from build123d import *

# Parameters (mm, degrees)
SKETCH_2_R          = 3
EXTRUDE_1_DEPTH     = 4
SKETCH_3_R          = 2
EXTRUDE_2_DEPTH     = 3
SKETCH_4_R          = 1
CUT_EXTRUDE_1_DEPTH = 10.110433579
SKETCH_5_R          = 3
EXTRUDE_3_DEPTH     = 2


with BuildPart() as part:
    # 草图2 → 凸台-拉伸1 (new body)
    with BuildSketch(Plane.XY):
        Circle(SKETCH_2_R)
    extrude(amount=EXTRUDE_1_DEPTH)

    # 草图3 → 凸台-拉伸2 (add)
    with BuildSketch(Plane.XY.offset(4)):
        Circle(SKETCH_3_R)
    extrude(amount=EXTRUDE_2_DEPTH)

    # 草图4 → 切除-拉伸1 (cut, through all)
    with BuildSketch(Plane(origin=(2, 0, 0), x_dir=(0, 0, -1), z_dir=(1, 0, 0))):
        with Locations(Location((-5.5, 0, 0), (0, 0, 180))):
            Circle(SKETCH_4_R)
    extrude(amount=-CUT_EXTRUDE_1_DEPTH, mode=Mode.SUBTRACT)

    # 草图5 → 凸台-拉伸3 (add)
    with BuildSketch(Plane.XY.offset(7)):
        Circle(SKETCH_5_R)
    extrude(amount=EXTRUDE_3_DEPTH)


solid = part.part
Source: CAD feature listing. Evaluate the final solid. Frame: model axes, mm. A direction names the side the tool comes from. Round coordinates to 2 decimals unless told otherwise and drop trailing zeros. Loops run counter-clockwise (first coordinate to the right, second up) from the corner with the lowest first, then second, coordinate; pieces in that order, holes last. Notation, with made-up numbers: (73, 2.25) - (123, 2.25) arc R14 cw to (123, 29.25) - close; hole circle Ø8 at (-28.5, 44.25). An arc over 180 degrees is marked (long way). Write item = value, one per line. Start each with the question number.
Item 1: Mould query, pull axis Y, two halves, no side actions, for faces 3 (the face through (1, -2, 4)), 4 (the face through (0.03, -0.84, 6.04)), 5 (the face through (-1.6, -1.2, 5.5)). Classes: released by +Y, released by -Y, zero draft, split by the parting line, or undercut.
Item 2: Section query A-A on x = 0. Output: boundary loops of the cut face in (y, z).
Item 3: Reachability of faces 1 (the face through (-3, 0, 8)), 2 (the face through (1, -2, 7)) from +Z, -Z, +X, -X, +Y, -Y: full face, straight path, thin tool, end or side. Return the list, or none.
Item 4: Section query C-C on x = 2.15. Output: boundary loops of the cut face in (y, z), plus the area to 3 significant figures.
Item 5: Section query D-D on y = -2.45. Output: boundary loops of the cut face in (x, z).
Item 6: Section query B-B on y = 0. Output: boundary loops of the cut face in (x, z).
Item 7: Material intervals for line 1 (Z direction, x = -1.9, y = 1.45); line 2 (Y direction, x = 0.1, z = 5.5); line 3 (Y direction, x = 0.8, z = 5.5), sorted ascending.
Results list:
q1.face_3 = zero draft
q1.face_4 = undercut
q1.face_5 = split by the parting line
q2.outline = (-3, 0) - (3, 0) - (3, 4) - (2, 4) - (2, 7) - (3, 7) - (3, 9) - (-3, 9) - (-3, 7) - (-2, 7) - (-2, 4) - (-3, 4) - close; hole circle Ø2 at (0, 5.5)
q3.face_1 = +Z, -Z
q3.face_2 = none
q4.outline = (-2.09, 0) - (2.09, 0) - (2.09, 4) - (-2.09, 4) - close; (-2.09, 7) - (2.09, 7) - (2.09, 9) - (-2.09, 9) - close
q4.area = 25.1 mm²
q5.outline = (-1.73, 0) - (1.73, 0) - (1.73, 4) - (-1.73, 4) - close; (-1.73, 7) - (1.73, 7) - (1.73, 9) - (-1.73, 9) - close
q6.outline = (-3, 0) - (3, 0) - (3, 4) - (2, 4) - (2, 4.5) - (-2, 4.5) - (-2, 4) - (-3, 4) - close; (-3, 7) - (-2, 7) - (-2, 6.5) - (2, 6.5) - (2, 7) - (3, 7) - (3, 9) - (-3, 9) - close
q7.line_1 = 0 to 4, 7 to 9
q7.line_2 = -2 to -1, 1 to 2
q7.line_3 = -1.83 to -1, 1 to 1.83
